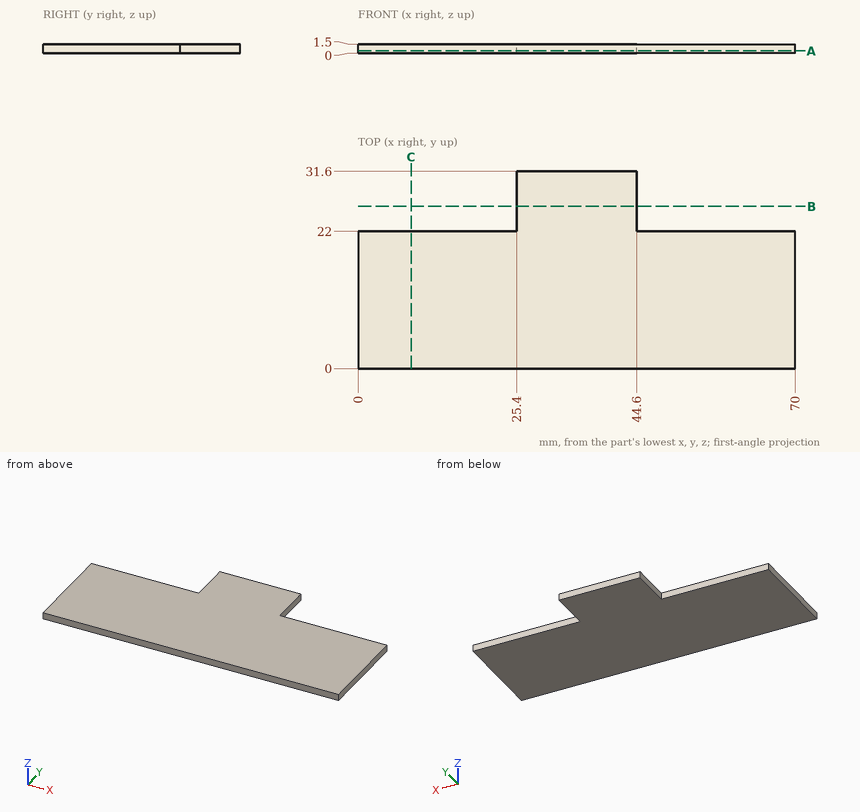
Could you check a few things on this drawing? It's one solid part, dimensions in mm from its lowest x, y, z. Give positions to 0.01 mm unless a question says otherwise; leave off trailing zeros. Order: outer loops, then holes, each group sorted by start corner. A loop starts at its lowest first (then second) coordinate and runs counter-clockwise, first axis right, second up. Notation, with made-up numbers: M 89.5,53.25 L 128.5,53.25 A33 cw 128.5,91.25 Z; hole C 84.5,35 d3. An arc over 180 degrees is marked long. Use one line per item in the form item = value.
Item 1: If we section it at B-B, the plane y = 26: Write out the boundary of the cut face in (x, z), and give its area (3 significant figures).
Values follow:
outline = M 25.4,0 L 44.6,0 L 44.6,1.5 L 25.4,1.5 Z
area = 28.8 mm^2
Item 2: If we section it at C-C, the plane x = 8.5: Write out the boundary of the cut face in (y, z).
Values follow:
outline = M 0,0 L 22,0 L 22,1.5 L 0,1.5 Z
Item 3: Will this pin go through, and if not, where does the flat tip stop? pin 1 Ø0.8 at (x, z) = (14, 0.5) entering from +Y.
Values follow:
pin_1 = 22
Item 4: If we section it at A-A, the plane z = 0.4: Write out the boundary of the cut face in (x, y).
Values follow:
outline = M 0,0 L 70,0 L 70,22 L 44.6,22 L 44.6,31.6 L 25.4,31.6 L 25.4,22 L 0,22 Z
Item 5: If I drill on line 1 along Y through (x, z) = (6.5, 0.1); line 2 along X through (y, z) = (30, 1.3), over which ranges is the centre line in solid material (lowest first)? Write a range as [from, to].
Values follow:
line_1 = [0, 22]
line_2 = [25.4, 44.6]
